```python
from build123d import *

# Parameters (mm, degrees)
HOUSING_DEPTH                      = 12.8
CUT_EXTRUDE_3_DEPTH                = 9.3
SKETCH_3_W                         = 4.1
SKETCH_3_H                         = 4.1
CUT_EXTRUDE_4_DEPTH                = 9.3
PATTERN_LINEAR_1_COUNT             = 2
PATTERN_LINEAR_1_PITCH             = 4.2
PATTERN_LINEAR_1_COUNT_DIR2        = 2
PATTERN_LINEAR_1_PITCH_DIR2        = 4.2
PATTERN_LINEAR_2_COUNT             = 2
PATTERN_LINEAR_2_PITCH             = 4.2
PATTERN_LINEAR_2_COUNT_DIR2        = 2
PATTERN_LINEAR_2_PITCH_DIR2        = 4.2
SKETCH_4_W                         = 1
SKETCH_4_H                         = 1
EXTRUDE_2286_DEPTH                 = 6
CHAMFER_1_SIZE                     = 0.5
PATTERN_LINEAR_3_COUNT             = 2
PATTERN_LINEAR_3_PITCH             = 4.2
CHAMFER_1_OF_PATTERN_LINEAR_3_SIZE = 0.5
EXTRUDE_START                      = -3.1
EXTRUDE_3473_DEPTH                 = 3.4
EXTRUDE_3845_DEPTH                 = 3.5
CUT_EXTRUDE_5_DEPTH                = 1.25
PATTERN_LINEAR_4_COUNT             = 2
PATTERN_LINEAR_4_PITCH             = 4.2


with BuildPart() as part:
    # Эскиз1 → Housing (new body)
    with BuildSketch(Plane(origin=(0, 0, 0), x_dir=(1, 0, 0), z_dir=(0, 1, 0))):
        with BuildLine():
            Line((-2.7, 4.2), (-2.7, -2.7))
            Line((-2.7, -2.7), (6.9, -2.7))
            Line((6.9, -2.7), (6.9, 6.9))
            Line((6.9, 6.9), (-2.7, 6.9))
            Line((-2.7, 6.9), (-2.7, 5))
            ThreePointArc((-2.7, 5), (-3.1, 4.6), (-2.7, 4.2))
        make_face()
    extrude(amount=HOUSING_DEPTH)

    # Эскиз2 → Вырез-Вытянуть3 (cut)
    with BuildSketch(Plane(origin=(0, 12.8, 0), x_dir=(1, 0, 0), z_dir=(0, 1, 0))):
        Polygon((-2.05, -2.05), (-2.05, 1.05), (-1.05, 2.05), (1.05, 2.05), (2.05, 1.05), (2.05, -2.05), align=None)
    cut_extrude_3 = extrude(amount=-CUT_EXTRUDE_3_DEPTH, mode=Mode.SUBTRACT)

    # Эскиз3 → Вырез-Вытянуть4 (cut)
    with BuildSketch(Plane(origin=(0, 12.8, 0), x_dir=(1, 0, 0), z_dir=(0, 1, 0))):
        with Locations((0, 4.2)):
            Rectangle(SKETCH_3_W, SKETCH_3_H)
    cut_extrude_4 = extrude(amount=-CUT_EXTRUDE_4_DEPTH, mode=Mode.SUBTRACT)

    # Линейный массив1: Cut-Extrude 4 2 × 2, 2 skipped
    with Locations(*[(i * PATTERN_LINEAR_1_PITCH, 0, j * PATTERN_LINEAR_1_PITCH_DIR2) for i in range(PATTERN_LINEAR_1_COUNT) for j in range(PATTERN_LINEAR_1_COUNT_DIR2) if (i, j) not in ((0, 0), (0, 1), (1, 0))]):
        add(cut_extrude_4, mode=Mode.SUBTRACT)

    # Линейный массив2: Cut-Extrude 3 2 × 2, 2 skipped
    with Locations(*[(i * PATTERN_LINEAR_2_PITCH, 0, -j * PATTERN_LINEAR_2_PITCH_DIR2) for i in range(PATTERN_LINEAR_2_COUNT) for j in range(PATTERN_LINEAR_2_COUNT_DIR2) if (i, j) not in ((0, 0), (0, 1), (1, 0))]):
        add(cut_extrude_3, mode=Mode.SUBTRACT)

    # Эскиз4 → Extrude 2286 (add)
    with BuildSketch(Plane(origin=(0, 3.5, 0), x_dir=(1, 0, 0), z_dir=(0, 1, 0))):
        Rectangle(SKETCH_4_W, SKETCH_4_H)
        with Locations((0, 4.2)):
            Rectangle(SKETCH_4_W, SKETCH_4_H)
    extrude_2286 = extrude(amount=EXTRUDE_2286_DEPTH)

    # Фаска1
    chamfer_1_edges = [part.edges().sort_by_distance(p)[0] for p in [
        (0.5, 9.5, 0),
        (0, 9.5, -0.5),
        (-0.5, 9.5, 0),
        (0, 9.5, 0.5),
        (0.5, 9.5, -4.2),
        (0, 9.5, -4.7),
        (-0.5, 9.5, -4.2),
        (0, 9.5, -3.7),
    ]]
    chamfer(chamfer_1_edges, length=CHAMFER_1_SIZE - 0.0001)  # a hair under: the kernel refuses the full size

    # Линейный массив3: Extrude 2286 ×2
    with Locations(*[(i * PATTERN_LINEAR_3_PITCH, 0, 0) for i in range(1, PATTERN_LINEAR_3_COUNT)]):
        add(extrude_2286)

    # Фаска1 of Линейный массив3
    chamfer_1_of_pattern_linear_3_edges = [part.edges().sort_by_distance(p)[0] for p in [
        (4.7, 9.5, 0),
        (4.2, 9.5, -0.5),
        (3.7, 9.5, 0),
        (4.2, 9.5, 0.5),
        (4.7, 9.5, -4.2),
        (4.2, 9.5, -4.7),
        (3.7, 9.5, -4.2),
        (4.2, 9.5, -3.7),
    ]]
    chamfer(chamfer_1_of_pattern_linear_3_edges, length=CHAMFER_1_OF_PATTERN_LINEAR_3_SIZE - 0.0001)  # a hair under: the kernel refuses the full size

    # Эскиз5 → Extrude 3473 (add)
    with BuildSketch(Plane.ZY.offset(2.7).offset(EXTRUDE_START)):
        Polygon((2.7, 9.6), (2.7, 12.8), (4.1, 10.375128869), (4.1, 9.6), align=None)
    extrude(amount=-EXTRUDE_3473_DEPTH)

    # Эскиз6 → Extrude 3845 (add)
    with BuildSketch(Plane.XZ):
        Polygon((-0.6, -4.55), (-0.6, -5.15), (0.6, -5.15), (0.6, -4.55), (0.5, -4.55), (0.5, -5.05), (-0.5, -5.05), (-0.5, -4.55), align=None)
        Polygon((-0.5, 0.35), (-0.6, 0.35), (-0.6, 0.95), (0.6, 0.95), (0.6, 0.35), (0.5, 0.35), (0.5, 0.85), (-0.5, 0.85), align=None)
    extrude_3845 = extrude(amount=EXTRUDE_3845_DEPTH)

    # Эскиз7 → Вырез-Вытянуть5 (cut)
    with BuildSketch(Plane(origin=(0.6, 0, 0), x_dir=(0, 0, -1), z_dir=(1, 0, 0))):
        Polygon((-0.65, -3.5), (-0.35, -2.5), (4.55, -2.5), (4.85, -3.5), align=None)
    cut_extrude_5 = extrude(amount=-CUT_EXTRUDE_5_DEPTH, mode=Mode.SUBTRACT)

    # Линейный массив4: Extrude 3845, Вырез-Вытянуть5 ×2
    with Locations(*[(i * PATTERN_LINEAR_4_PITCH, 0, 0) for i in range(1, PATTERN_LINEAR_4_COUNT)]):
        add(extrude_3845)
        add(cut_extrude_5, mode=Mode.SUBTRACT)


solid = part.part
```
Could you check a few things on this model? Use its own coordinates, in mm. A direction names the side the tool comes from. Round coordinates to 2 decimals unless told otherwise and drop trailing zeros. Loops run counter-clockwise (first coordinate to the right, second up) from the corner with the lowest first, then second, coordinate; pieces in that order, holes last. Notation, with made-up numbers: M 10,53.25 L 15,53.25 A34 cw 15,88.25 Z; hole C 10.25,-28.5 d10. An arc over 180 degrees is marked long. Answer as CSV lines item,"result".
1) Imagine slicing it at A-A on x = 1.75. List the corners of the cut face in (y, z) for me.
From the geometry:
outline,"M 0,-6.9 L 12.8,-6.9 L 12.8,-6.25 L 3.5,-6.25 L 3.5,-2.15 L 12.8,-2.15 L 12.8,-1.35 L 3.5,-1.35 L 3.5,2.05 L 12.8,2.05 L 12.8,2.7 L 10.38,4.1 L 9.6,4.1 L 9.6,2.7 L 0,2.7 Z"
2) If I drill on probe 1 along X at (y, z) = (8.75, -1.5); probe 2 along Z at (x, y) = (-1.75, 4.25); probe 3 along Z at (x, y) = (-2, 5.25), over which ranges is the centre line in solid material (lowest first)?
From the geometry:
probe 1,"-2.7 to -1.6, 1.6 to 2.15, 6.25 to 6.9"
probe 2,"-6.9 to -6.25, -2.15 to -1.35, 2.05 to 2.7"
probe 3,"-6.9 to -6.25, -2.15 to -1.1, 2.05 to 2.7"
3) Imagine slicing it at C-C on y = 2.75. List the corners of the cut face in (x, z) for me, and give its area (3 significant figures).
From the geometry:
outline,"M -2.7,-6.9 L 6.9,-6.9 L 6.9,2.7 L -2.7,2.7 L -2.7,-4.2 A0.4 ccw -2.7,-5 Z"
area,"92.4 mm^2"
4) We'd pull the mould along X, two halves only. Please class faces 4 (the flat face through (1.8, 12.8, -6.4)), 5 (the flat face through (6.9, 6, -2)), 6 (the flat face through (3.7, 6, -4)): released by +X, released by -X, zero draft, split by the parting line, or undercut.
From the geometry:
face 4,"zero draft"
face 5,"released by +X"
face 6,"undercut"
5) Which directions (+Z, -Z, +X, -X, +Y, -Y) give clear straight access to the entire face, cutting with the end or side of a thin tool? Please do faces 1 (the flat face through (3.8, 11, 3)), 2 (the flat face through (0.5, 6, -4)), 3 (the flat face through (-2.7, 6, -1)).
From the geometry:
face 1,"+Z, +X, +Y, -Y"
face 2,"+Y"
face 3,"+Z, -X, +Y, -Y"
6) Imagine slicing it at B-B on z = -6. List the corners of the cut face in (x, y) for me, and give its area (3 significant figures).
From the geometry:
outline,"M -2.7,0 L 6.9,0 L 6.9,12.8 L 5.5,12.8 L 5.5,3.5 L 2.9,3.5 L 2.9,12.8 L 2.05,12.8 L 2.05,3.5 L -2.05,3.5 L -2.05,12.8 L -2.7,12.8 Z"
area,"60.6 mm^2"
7) Imagine slicing it at D-D on x = -1.25. List the corners of the cut face in (y, z) for me, and give its area (3 significant figures).
From the geometry:
outline,"M 0,-6.9 L 12.8,-6.9 L 12.8,-6.25 L 3.5,-6.25 L 3.5,-2.15 L 12.8,-2.15 L 12.8,-1.85 L 3.5,-1.85 L 3.5,2.05 L 12.8,2.05 L 12.8,2.7 L 0,2.7 Z"
area,"48.5 mm^2"
8) For pin 1 Ø1.1 at (x, y) = (0, -1.5) entering from +Z; pin 2 Ø5 at (x, z) = (0, -2.5) entering from -Y; pin 3 Ø1 at (y, z) = (8.5, -6) entering from -X; pin 4 Ø0.6 at (x, y) = (4.5, -1.5) entering from -Z, each with a flat end and sliding along its axis, tell me the tip position at first contact or that it passes through.
From the geometry:
pin 1,"z = 0.95"
pin 2,"y = -3.5"
pin 3,"x = -2.7"
pin 4,"z = -5.15"
